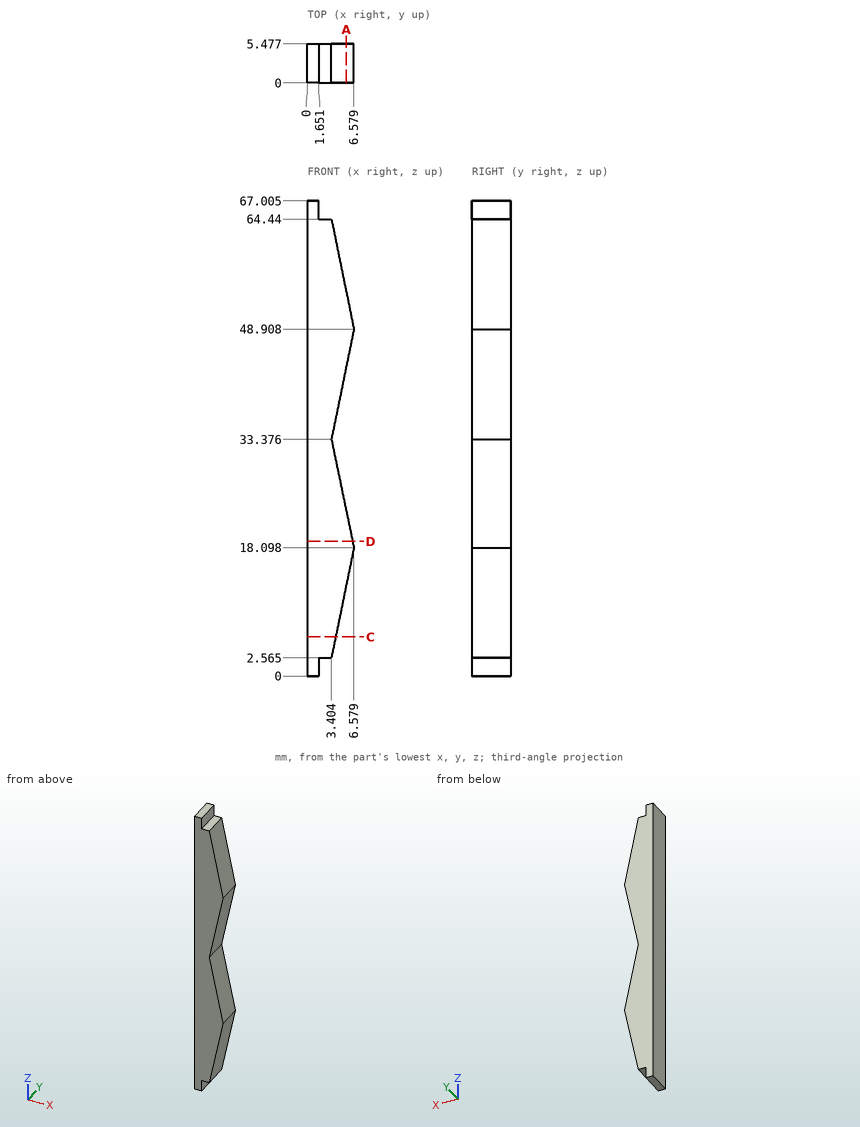
Print and shaded views of the part. All mm, measured from the part's lowest x, y and z. Round coordinates to 2 decimals unless told otherwise and drop trailing zeros. Write each loop counter-clockwise with the first axis right and the second up, starting at its lowest first coordinate (ties: lowest second). Pieces come first, ordered by that corner, then holes. Notation, with made-up numbers: M 35.25,81 L 89.25,81 A30 ccw 89.25,103 Z; hole C 0.5,-19.75 d3. An arc over 180 degrees is marked long. Use a Markdown table: item, result. Add a question column.
1. Slice it at A-A on x = 5.5. Give the cut face in (y, z) (1 decimal), then the cut area to 3 significant figures.
2. Drill centre lines: probe 1 along Z at (x, y) = (3, 2.4) (1 decimal); probe 2 along X at (y, z) = (2.85, 36.5); probe 3 along X at (y, z) = (4.9, 32.5) (1 decimal). Where is each one in solid material? Low to high.
3. Slice it at D-D on z = 19. Give the cut face in (x, y), then the cut area to 3 significant figures.
4. Flat gauge pins, fed straight in: P1, Ø0.8, axis at y = 1.5, z = 0.5, coming from the +X side; P2, Ø0.9, axis at x = 2.5, y = 3.5, coming from the +Z side. Where does each tip first touch, or does it go through?
5. Slice it at C-C on z = 5.5. Give the cut face in (x, y).
Reply:
| question | item | result |
|---|---|---|
| 1 | outline | M 0,12.8 L 5.5,12.8 L 5.5,23.3 L 0,23.3 Z; M 0,43.6 L 5.5,43.6 L 5.5,54.2 L 0,54.2 Z |
| 1 | area | 115 mm^2 |
| 2 | probe 1 | z = 2.6 to 64.4 |
| 2 | probe 2 | x = 0 to 4.04 |
| 2 | probe 3 | x = 0 to 3.6 |
| 3 | outline | M 0,0 L 6.39,0 L 6.39,5.48 L 0,5.48 Z |
| 3 | area | 35.0 mm^2 |
| 4 | P1 | stops at x = 1.65 |
| 4 | P2 | stops at z = 64.44 |
| 5 | outline | M 0,0 L 4,0 L 4,5.48 L 0,5.48 Z |
